```python
from build123d import *

# Parameters (mm, degrees)
SKETCH1_W               = 50.8
SKETCH1_H               = 25.4
SKETCH1_W_2             = 45.72
SKETCH1_H_2             = 20.32
EXTRUDE_THIN1_DEPTH     = 163.5125
SKETCH3_R               = 2.4765
CUT_EXTRUDE2_DEPTH      = 13.7
CUT_EXTRUDE2_DEPTH_BACK = 13.7
SKETCH4_R               = 2.4765
CUT_EXTRUDE3_DEPTH      = 2.54


with BuildPart() as part:
    # Sketch1 → Extrude-Thin1 (new body, symmetric)
    with BuildSketch(Plane(origin=(0, 0, 0), x_dir=(1, 0, 0), z_dir=(0, 1, 0))):
        Rectangle(SKETCH1_W, SKETCH1_H)
        Rectangle(SKETCH1_W_2, SKETCH1_H_2, mode=Mode.SUBTRACT)
    extrude(amount=EXTRUDE_THIN1_DEPTH, both=True)

    # Sketch3 → Cut-Extrude2 (cut, two sides)
    with BuildSketch(Plane.XY) as cut_extrude2_sk:
        with Locations((-12.7, -125.4125)):
            Circle(SKETCH3_R)
        with Locations((12.7, -125.4125)):
            Circle(SKETCH3_R)
        with Locations((12.7, -150.8125)):
            Circle(SKETCH3_R)
        with Locations((-12.7, -150.8125)):
            Circle(SKETCH3_R)
        with Locations((12.7, 150.8125)):
            Circle(SKETCH3_R)
        with Locations((12.7, 125.4125)):
            Circle(SKETCH3_R)
        with Locations((-12.7, 125.4125)):
            Circle(SKETCH3_R)
        with Locations((-12.7, 150.8125)):
            Circle(SKETCH3_R)
    extrude(amount=CUT_EXTRUDE2_DEPTH, mode=Mode.SUBTRACT)
    extrude(cut_extrude2_sk.sketch, amount=-CUT_EXTRUDE2_DEPTH_BACK, mode=Mode.SUBTRACT)

    # Sketch4 → Cut-Extrude3 (cut)
    with BuildSketch(Plane(origin=(25.4, 0, 0), x_dir=(0, 0, -1), z_dir=(1, 0, 0))):
        with Locations((0, -46.0375)):
            Circle(SKETCH4_R)
        with Locations((0, -122.2375)):
            Circle(SKETCH4_R)
    extrude(amount=-CUT_EXTRUDE3_DEPTH, mode=Mode.SUBTRACT)


solid = part.part
```
Read the model definition and answer for the solid it produces. Units are mm, in the model's axes. A direction names the side the tool comes from. Coordinates: 2 decimals unless noted, no trailing zeros. Loops run counter-clockwise (first coordinate to the right, second up) from the corner with the lowest first, then second, coordinate; pieces in that order, holes last.
(1) A tool of negligible diameter and unlimited length cuts with its end or side. For faces 4 (the face through (-25.4, 2, 0)), 5 (the face through (-22.86, 2, 0)), from which of +Z, -Z, +X, -X, +Y, -Y can it reach the whole face along a straight path? Write none if from no direction.
Solution:
face 4: +Z, -Z, -X, +Y, -Y
face 5: +Y, -Y
(2) The part is cut by section A-A (x = -0.5). Determine the outline of the cut face in (y, z), and give its area (3 significant figures).
Solution:
outline: (-163.51, -12.7) - (163.51, -12.7) - (163.51, -10.16) - (-163.51, -10.16) - close; (-163.51, 10.16) - (163.51, 10.16) - (163.51, 12.7) - (-163.51, 12.7) - close
area: 1,660 mm2
(3) A flat-ended cylindrical pin translates along its axis: pin 1 Ø6.5 at (x, y) = (-12.7, -150.81) entering from -Z. Find the tip coordinate at first contact, or state that the pin passes through.
Solution:
pin 1: stops at z = -12.7
(4) The part is cut by section C-C (z = -5.5). Determine the outline of the cut face in (x, y), and give its area (3 significant figures).
Solution:
outline: (-25.4, -163.51) - (-22.86, -163.51) - (-22.86, 163.51) - (-25.4, 163.51) - close; (22.86, -163.51) - (25.4, -163.51) - (25.4, 163.51) - (22.86, 163.51) - close
area: 1,660 mm2
(5) The mould has two halves that part along Z. Classify faces 1 (the face through (0, 2, -12.7)), 2 (the face through (22.86, 2, 0)), 3 (the face through (25.4, 2, 0)): released by +Z, released by -Z, zero draft, split by the parting line, or undercut.
Solution:
face 1: released by -Z
face 2: undercut
face 3: zero draft
(6) Consider line 1 along Y through (x, z) = (24.05, 0); line 2 along Y through (x, z) = (-12.7, -11.2); line 3 along Z through (x, y) = (11.5, -60.5). Determine where each line is inside the solid, lowest interval first.
Solution:
line 1: y = -163.51 to -124.71, -119.76 to -48.51, -43.56 to 163.51
line 2: y = -163.51 to -153.29, -148.34 to -127.89, -122.94 to 122.94, 127.89 to 148.34, 153.29 to 163.51
line 3: z = -12.7 to -10.16, 10.16 to 12.7
(7) The part is cut by section B-B (y = -39.5). Determine the outline of the cut face in (x, z), and give its area (3 significant figures).
Solution:
outline: (-25.4, -12.7) - (25.4, -12.7) - (25.4, 12.7) - (-25.4, 12.7) - close; hole (-22.86, -10.16) - (22.86, -10.16) - (22.86, 10.16) - (-22.86, 10.16) - close
area: 361 mm2
